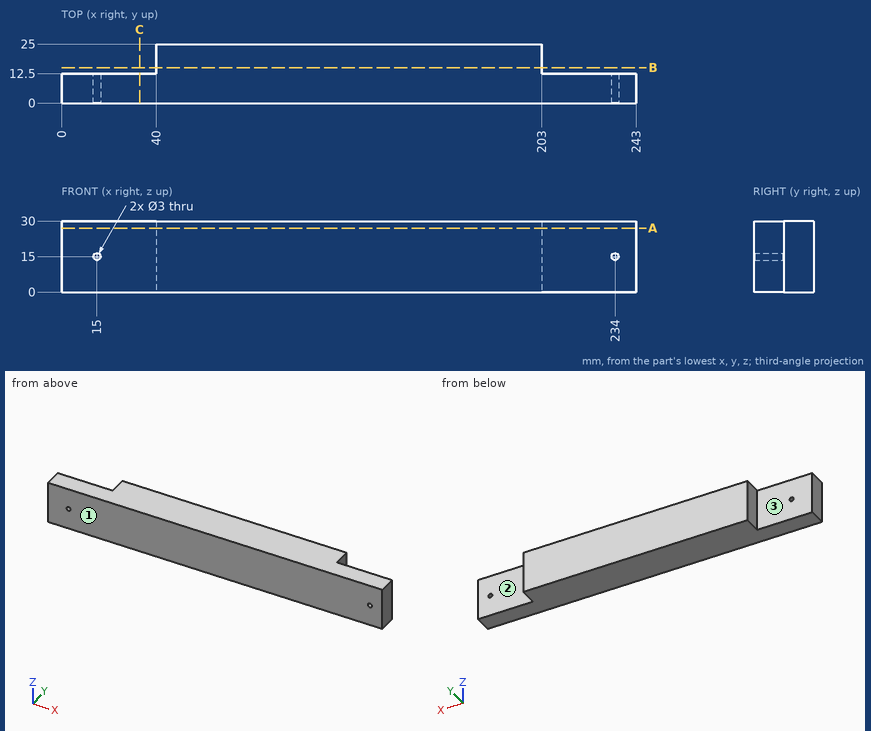
Geometry check sheet. Reference: drawing and pictorial views, mm from the part's lowest x, y, z. A direction names the side the tool comes from. Round coordinates to 2 decimals unless told otherwise and drop trailing zeros. Order: outer loops, then holes, each group sorted by start corner. A loop starts at its lowest first (then second) coordinate and runs counter-clockwise, first axis right, second up.
Q1. Cross-section at B-B, the plane y = 15. Enter the section's corners in (x, z), plus the area to 3 significant figures.
Filled sheet:
outline: (40, 0) - (203, 0) - (203, 30) - (40, 30) - close
area: 4,890 mm2
Q2. Set-up check for the marked faces 1, 2 and 3: record each of +Z, -Z, +X, -X, +Y, -Y from which the full face is reachable in a straight line by a thin tool's end or side.
Filled sheet:
face 1: +Z, -Z, +X, -X, -Y
face 2: +Z, -Z, +X, +Y
face 3: +Z, -Z, -X, +Y
Q3. Scan lines: L1, parallel to X at y = 8.5, z = 15; L2, parallel to Z at x = 15, y = 8.25; L3, parallel to X at y = 22, z = 6.5. Record each from-to range of solid material in increasing order.
Filled sheet:
L1: x = 0 to 13.5, 16.5 to 232.5, 235.5 to 243
L2: z = 0 to 13.5, 16.5 to 30
L3: x = 40 to 203
Q4. Cross-section at C-C, the plane x = 33. Enter the section's corners in (y, z).
Filled sheet:
outline: (0, 0) - (12.5, 0) - (12.5, 30) - (0, 30) - close
Q5. Depth check by flat-ended pin: P1, Ø1.5, axis at x = 111, y = 5, coming from the -Z side; P2, Ø1.8, axis at x = 15, z = 15, coming from the -Y side; P3, Ø6, axis at y = 16.5, z = 19.5, coming from the -X side; P4, Ø4, axis at x = 213, z = 18.5, coming from the +Y side. Enter the tip coordinate at first touch or a pass-through.
Filled sheet:
P1: stops at z = 0
P2: passes through
P3: stops at x = 40
P4: stops at y = 12.5
Q6. Cross-section at A-A, the plane z = 27. Enter the section's corners in (x, y), plus the area to 4 significant figures.
Filled sheet:
outline: (0, 0) - (243, 0) - (243, 12.5) - (203, 12.5) - (203, 25) - (40, 25) - (40, 12.5) - (0, 12.5) - close
area: 5,075 mm2
